```python
from build123d import *

# Parameters (mm, degrees)
EXTRUDE_1_DEPTH     = 10
CUT_EXTRUDE_1_REACH = 177.427
SKETCH_2_R          = 2.2
FILLET_1_R          = 0.6
SKETCH_3_W          = 10.144437824
SKETCH_3_H          = 10
EXTRUDE_2_DEPTH     = 15
CUT_EXTRUDE_2_REACH = 164.61
SKETCH_4_R          = 3.8
FILLET_2_R          = 3


with BuildPart() as part:
    # 草图1 → 凸台-拉伸1 (new body)
    with BuildSketch(Plane(origin=(0, 0, 0), x_dir=(1, 0, 0), z_dir=(0, 1, 0))):
        with BuildLine():
            Line((-19, 0), (19, 0))
            Line((19, 0), (44.854614973, 30.81233028))
            ThreePointArc((44.854614973, 30.81233028), (46.529317931, 33.929104052), (46.82231051, 37.455159084))
            Line((46.82231051, 37.455159084), (33.389549678, 146.856216784))
            ThreePointArc((33.389549678, 146.856216784), (34.753999407, 148.533855984), (36.376927445, 147.104765038))
            ThreePointArc((36.376927445, 147.104765038), (36.892496808, 144.296291333), (37.320815542, 141.473193853))
            Line((37.320815542, 141.473193853), (37.815132232, 139.258398169))
            ThreePointArc((37.815132232, 139.258398169), (37.817176658, 139.245056143), (37.817405692, 139.231560332))
            Line((37.817405692, 139.231560332), (37.557917484, 134.104765038))
            ThreePointArc((37.557917484, 134.104765038), (40.754926912, 130.959847465), (43.503129215, 134.503681536))
            Line((43.503129215, 134.503681536), (43.077003941, 137.813685213))
            Line((43.077003941, 137.813685213), (42.807637334, 138.925557366))
            ThreePointArc((42.807637334, 138.925557366), (42.806315787, 138.931905108), (42.80540838, 138.938325149))
            Line((42.80540838, 138.938325149), (42.129277547, 145.175318139))
            Line((42.129277547, 145.175318139), (41.965181023, 146.44996701))
            ThreePointArc((41.965181023, 146.44996701), (43.130662006, 148.010841711), (44.727999785, 146.895858405))
            Line((44.727999785, 146.895858405), (66.016482503, 37.376109146))
            ThreePointArc((66.016482503, 37.376109146), (66.063066684, 33.817543133), (64.860464706, 30.468019192))
            Line((64.860464706, 30.468019192), (38.23055697, -15.656334008))
            ThreePointArc((38.23055697, -15.656334008), (35.050772773, -18.836118205), (30.707106781, -20))
            Line((30.707106781, -20), (5.707106781, -20))
            Line((5.707106781, -20), (-5.707106781, -20))
            Line((-5.707106781, -20), (-25.399802658, -20))
            ThreePointArc((-25.399802658, -20), (-30.087775174, -18.833058003), (-33.681629288, -15.604582738))
            Line((-33.681629288, -15.604582738), (-64.860464706, 30.468019192))
            ThreePointArc((-64.860464706, 30.468019192), (-66.063066684, 33.817543133), (-66.016482503, 37.376109146))
            Line((-66.016482503, 37.376109146), (-46.829620455, 141.890886738))
            ThreePointArc((-46.829620455, 141.890886738), (-43.465252598, 152.148967586), (-37.480163066, 161.13372674))
            ThreePointArc((-37.480163066, 161.13372674), (-33.620696298, 161.680216975), (-32.479267504, 157.953116813))
            ThreePointArc((-32.479267504, 157.953116813), (-35.579400499, 146.14570295), (-34.973851142, 133.953116813))
            Line((-34.973851142, 133.953116813), (-47.176674229, 34.569098196))
            ThreePointArc((-47.176674229, 34.569098196), (-47.109221395, 33.75732882), (-46.723670812, 33.03978429))
            Line((-46.723670812, 33.03978429), (-19, 0))
        make_face()
    extrude(amount=EXTRUDE_1_DEPTH)

    # 草图2 → 切除-拉伸1 (cut, up to next)
    with BuildSketch(Plane(origin=(0, 10, 0), x_dir=(1, 0, 0), z_dir=(0, 1, 0)), mode=Mode.PRIVATE) as cut_extrude_1_sk1:
        with Locations(Location((0, -10, 0), (0, 0, 270))):
            Circle(SKETCH_2_R)
    cut_extrude_1_tool1 = extrude(cut_extrude_1_sk1.sketch, amount=-CUT_EXTRUDE_1_REACH, mode=Mode.PRIVATE) & part.part
    # 草图2 → 切除-拉伸1 (cut, up to next)
    with BuildSketch(Plane(origin=(0, 10, 0), x_dir=(1, 0, 0), z_dir=(0, 1, 0)), mode=Mode.PRIVATE) as cut_extrude_1_sk2:
        with Locations(Location((-26, -10, 0), (0, 0, 270))):
            Circle(SKETCH_2_R)
    cut_extrude_1_tool2 = extrude(cut_extrude_1_sk2.sketch, amount=-CUT_EXTRUDE_1_REACH, mode=Mode.PRIVATE) & part.part
    # 草图2 → 切除-拉伸1 (cut, up to next)
    with BuildSketch(Plane(origin=(0, 10, 0), x_dir=(1, 0, 0), z_dir=(0, 1, 0)), mode=Mode.PRIVATE) as cut_extrude_1_sk3:
        with Locations(Location((26, -10, 0), (0, 0, 270))):
            Circle(SKETCH_2_R)
    cut_extrude_1_tool3 = extrude(cut_extrude_1_sk3.sketch, amount=-CUT_EXTRUDE_1_REACH, mode=Mode.PRIVATE) & part.part
    # 草图2 → 切除-拉伸1 (cut, up to next)
    with BuildSketch(Plane(origin=(0, 10, 0), x_dir=(1, 0, 0), z_dir=(0, 1, 0)), mode=Mode.PRIVATE) as cut_extrude_1_sk4:
        with BuildLine():
            Line((-36.549558395, 121.120011078), (-38.607748185, 104.35740041))
            ThreePointArc((-38.607748185, 104.35740041), (-42.47341142, 116.594845153), (-44.332546284, 129.292956179))
            Line((-44.332546284, 129.292956179), (-43.845113062, 129.987442667))
            ThreePointArc((-43.845113062, 129.987442667), (-43.702378092, 130.509625408), (-43.924830211, 131.003146575))
            Line((-43.924830211, 131.003146575), (-44.447419993, 131.543571067))
            ThreePointArc((-44.447419993, 131.543571067), (-44.482588605, 132.737575539), (-44.499925482, 133.931972015))
            ThreePointArc((-44.499925482, 133.931972015), (-41.418283025, 136.952003662), (-38.505677682, 133.768634142))
            ThreePointArc((-38.505677682, 133.768634142), (-38.556072369, 132.542586282), (-38.556286633, 131.315503182))
            Line((-38.556286633, 131.315503182), (-38.546052546, 131.325051295))
            ThreePointArc((-38.546052546, 131.325051295), (-38.780683801, 130.91622187), (-38.744387532, 130.446247504))
            Line((-38.744387532, 130.446247504), (-38.486748585, 129.793872308))
            ThreePointArc((-38.486748585, 129.793872308), (-37.841140795, 125.384806825), (-36.549558395, 121.120011078))
        make_face()
    cut_extrude_1_tool4 = extrude(cut_extrude_1_sk4.sketch, amount=-CUT_EXTRUDE_1_REACH, mode=Mode.PRIVATE) & part.part
    add(cut_extrude_1_tool1.solids().sort_by_distance((0, 10, 10))[0], mode=Mode.SUBTRACT)
    add(cut_extrude_1_tool2.solids().sort_by_distance((-26, 10, 10))[0], mode=Mode.SUBTRACT)
    add(cut_extrude_1_tool3.solids().sort_by_distance((26, 10, 10))[0], mode=Mode.SUBTRACT)
    add(cut_extrude_1_tool4.solids().sort_by_distance((-40.502089, 10, -123.156617))[0], mode=Mode.SUBTRACT)

    # 圆角1
    fillet_1_edges = [part.edges().sort_by_distance(p)[0] for p in [
        (-36.549558395, 5, -121.120011078),
        (-34.973851142, 5, -133.953116813),
    ]]
    fillet(fillet_1_edges, radius=FILLET_1_R)

    # 草图3 → 凸台-拉伸2 (add)
    with BuildSketch(Plane(origin=(70.613618069, 0, -13.725896909), x_dir=(-0.19080899537654988, 0, -0.9816271834476631), z_dir=(0.9816271834476631, 0, -0.19080899537654988))):
        with Locations((29.616052291, 5)):
            Rectangle(SKETCH_3_W, SKETCH_3_H)
    extrude(amount=EXTRUDE_2_DEPTH)

    # 草图4 → 切除-拉伸2 (cut, up to next)
    with BuildSketch(Plane(origin=(-4.68318419, 0, -24.092894031), x_dir=(0.981627183447663, 0, -0.19080899537654997), z_dir=(0.19080899537654997, 0, 0.981627183447663)), mode=Mode.PRIVATE) as cut_extrude_2_sk1:
        with Locations((79.435271618, 5)):
            Circle(SKETCH_4_R)
    cut_extrude_2_tool1 = extrude(cut_extrude_2_sk1.sketch, amount=-CUT_EXTRUDE_2_REACH, mode=Mode.PRIVATE) & part.part
    add(cut_extrude_2_tool1.solids().sort_by_distance((73.292638, 5, -39.249858))[0], mode=Mode.SUBTRACT)

    # 圆角2
    fillet_2_edges = [part.edges().sort_by_distance(p)[0] for p in [
        (79.687016636, 0, -45.659953836),
        (79.687016636, 10, -45.659953836),
    ]]
    fillet(fillet_2_edges, radius=FILLET_2_R)


solid = part.part
```
Design review of the part built by this model. Coordinates are the model's own, in mm. A direction names the side the tool comes from. Coordinates: 2 decimals unless noted, no trailing zeros. Order: outer loops, then holes, each group sorted by start corner. A loop starts at its lowest first (then second) coordinate and runs counter-clockwise, first axis right, second up. Notation, with made-up numbers: (28.5, -16.75) - (36.5, -16.75) arc R11 cw to (36.5, -10.75) - close; hole circle Ø7 at (11.5, -22.75). An arc over 180 degrees is marked (long way). Answer in a Markdown table with one row per item.
(1) Wall thickness on line 1 along X through (y, z) = (2.5, -128); line 2 along X through (y, z) = (5, -126); line 3 along X through (y, z) = (4.5, 10): over which ranges is each line inside the solid? List them lowest first. Write a range as from..to.
Checked values:
| item | result |
|---|---|
| line 1 | -49.38..-44.24, -38.3..-35.7, 35.7..48.4 |
| line 2 | -49.75..-44.05, -37.97..-35.95, 35.95..48.79 |
| line 3 | -37.47..-28.2, -23.8..-2.2, 2.2..23.8, 28.2..41.5 |
(2) The part is to be moulded in two halves that separate along X. For faces 4 (the cylindrical face through (-33.67, 4.93, -161.71)), 5 (the flat face through (-47, 10, -51)), 6 (the cylindrical face through (23.852, 5.07, 9.523)), say which applies: released by +X, released by -X, zero draft, split by the parting line, or undercut.
Checked values:
| item | result |
|---|---|
| face 4 | split by the parting line |
| face 5 | zero draft |
| face 6 | undercut |
(3) For faces 1 (the flat face through (0, 5, 0)), 2 (the cylindrical face through (78.79, 0.86, -45.56)), 3 (the cylindrical face through (46.515, 4.93, -33.881)), list the 3-axis set-ups (+Z, -Z, +X, -X, +Y, -Y) from which the entire face can be reached by the end or side of a thin tool; tool diameter is ignored.
Checked values:
| item | result |
|---|---|
| face 1 | -Z, +Y, -Y |
| face 2 | -Z, +X, -Y |
| face 3 | +Y, -Y |
(4) Clearance check with flat-ended pins moving along their axes: pin 1 (8 mm diameter, centred on x = 40.55, z = -133.95, fed in from +Y); pin 2 (6 mm diameter, centred on x = -28, y = 1.5, fed in from -Z); pin 3 (4 mm diameter, centred on y = 1.5, z = -17, fed in from +X); pin 4 (3 mm diameter, centred on x = -42.5, y = 1.5, fed in from +Z). State where each tip first meets the part, or that it passes through.
Checked values:
| item | result |
|---|---|
| pin 1 | y = 10 |
| pin 2 | z = -14.3 |
| pin 3 | x = 58.24 |
| pin 4 | z = 4.79 |
(5) Consider section D-D on z = -85.5. State the section outline as (x, y) points, plus the area to 3 significant figures.
Checked values:
| item | result |
|---|---|
| outline | (-57.18, 0) - (-40.92, 0) - (-40.92, 10) - (-57.18, 10) - close; (40.92, 0) - (56.66, 0) - (56.66, 10) - (40.92, 10) - close |
| area | 320 mm^2 |
(6) Consider section B-B on z = 10. State the section outline as (x, y) points, plus the area to 3 significant figures.
Checked values:
| item | result |
|---|---|
| outline | (-37.47, 0) - (-28.2, 0) - (-28.2, 10) - (-37.47, 10) - close; (-23.8, 0) - (-2.2, 0) - (-2.2, 10) - (-23.8, 10) - close; (2.2, 0) - (23.8, 0) - (23.8, 10) - (2.2, 10) - close; (28.2, 0) - (41.5, 0) - (41.5, 10) - (28.2, 10) - close |
| area | 658 mm^2 |
(7) Consider section A-A on x = 0. State the section outline as (y, z) points, plus the area to 3 significant figures.
Checked values:
| item | result |
|---|---|
| outline | (0, 0) - (10, 0) - (10, 7.8) - (0, 7.8) - close; (0, 12.2) - (10, 12.2) - (10, 20) - (0, 20) - close |
| area | 156 mm^2 |
(8) Consider section C-C on x = -41.5. State the section outline as (y, z) points, plus the area to 3 significant figures.
Checked values:
| item | result |
|---|---|
| outline | (0, -155.72) - (10, -155.72) - (10, -136.95) - (0, -136.95) - close; (0, -112.79) - (10, -112.79) - (10, -80.8) - (0, -80.8) - close; (0, -26.81) - (10, -26.81) - (10, 4.05) - (0, 4.05) - close |
| area | 816 mm^2 |
